Autodesk Inventor part; units mm, degrees
ref_plane "YZ Plane" through (0, 0, 0) normal (1, 0, 0) x (0, 1, 0)
ref_plane "XZ Plane" through (0, 0, 0) normal (0, 1, 0) x (-1, 0, 0)
ref_plane "XY Plane" through (0, 0, 0) normal (0, 0, 1) x (1, 0, 0)
sketch "Sketch1" plane through (0, 0, 0) normal (0, 0, 1) x (1, 0, 0)
  line L0 (63.5, 76.2) -> (0, 76.2)
  line L1 (0, 76.2) -> (0, 53.975)
  circle A0 centre (31.75, 47.625) radius 4.05
  line L2 (19.05, -6.35) -> (44.45, -6.35)
  line L3 (63.5, 53.975) -> (63.5, 76.2)
  line L4 (31.75, 76.2) -> (31.75, -6.35)
  circle A1 centre (31.75, 12.7) radius 2.6543
  circle A2 centre (31.75, -12.7) radius 2.6543
  circle A3 centre (31.75, -38.1) radius 2.6604
  line L5 (63.5, 53.975) -> (63.5, -6.35)
  line L6 (63.5, -6.35) -> (0, -6.35)
  line L7 (0, -6.35) -> (0, 53.975)
  line L8 (19.05, -15.3543) -> (19.05, -51.598)
  line L9 (19.05, -51.598) -> (44.45, -51.598)
  line L10 (44.45, -51.598) -> (44.45, -15.3543)
  line L11 (63.5, 53.975) -> (44.45, -15.3543)
  line L12 (0, 53.975) -> (19.05, -15.3543)
  point P0 (0, 0)
  dimension "d0" = 63.5
  dimension "d2" = 8.1
  dimension "d5" = 28.575
  dimension "d50" = 82.55
  dimension "d54" = 5.3086
  dimension "d55" = 63.5
  dimension "d59" = 25.4
  dimension "d60" = 25.4
  dimension "d61" = 25.4
extrude "Extrusion1" add sketch "Sketch1" along normal blind 3.302 contours L3 L11 L6 L2 L4 A1 A0 L0 | L4 A0 A1 L2 L6 L12 L1 L0 | L11 L10 L9 L8 L12 L6 L2
fillet "Fillet11" radius 17.78 1 edges at (63.5, 76.2, 1.651)
fillet "Fillet12" radius 17.78 1 edges at (0, 76.2, 1.651)
sketch "Sketch3" plane through (0, 0, 3.302) normal (0, 0, 1) x (1, 0, 0)
  circle A0 centre (31.75, 47.625) radius 4.05
  circle A1 centre (31.75, 47.625) radius 16
  circle A2 centre (31.75, 47.625) radius 8
  circle A3 centre (31.75, 47.625) radius 12
  line L0 (31.75, 47.625) -> (31.75, 69.8383)
  line L1 (31.75, 47.625) -> (53.9633, 47.625) construction
  point P0 (0, 0)
  point P1 (31.75, 59.625)
  dimension "d28" = 24
  dimension "d26" = 32
  dimension "d27" = 16
  dimension "d36" = 90
hole "Hole1" at (31.75, 59.625, 3.302) direction (0, 0, -1) diameter 4.4958 depth 14.1986 tip angle 118
pattern_circular "Circular Pattern1" count 4 over 360 about axis through (31.75, 47.625, 0) along (0, 0, 1) of "Hole1"
sketch "Sketch4" plane through (0, 0, 3.302) normal (0, 0, 1) x (1, 0, 0)
  circle A0 centre (31.75, 47.625) radius 4.05
  circle A1 centre (31.75, 47.625) radius 12
  circle A2 centre (31.75, 47.625) radius 16
  circle A3 centre (31.75, 47.625) radius 20.955
  line L0 (45.72, 76.2) -> (17.78, 76.2)
  line L1 (31.75, 47.625) -> (51.1677, 67.0427)
  line L2 (31.75, 47.625) -> (59.2107, 47.625) construction
  point P0 (0, 0)
  point P1 (46.5674, 62.4424)
  dimension "d42" = 41.91
  dimension "d40" = 24
  dimension "d41" = 32
  dimension "d58" = 45
hole "Hole2" at (46.5674, 62.4424, 3.302) direction (0, 0, -1) diameter 5.1054 depth 16.256 tip angle 118
pattern_circular "Circular Pattern2" count 4 over 360 about axis through (31.75, 47.625, 0) along (0, 0, 1) of "Hole2"
fillet "Fillet16" radius 6.35 2 edges at (44.45, -15.3543, 1.651) (19.05, -15.3543, 1.651)
sketch "Sketch5" plane through (0, 0, 3.302) normal (0, 0, 1) x (1, 0, 0)
  circle A0 centre (31.75, 47.625) radius 4.05
  circle A1 centre (31.75, 47.625) radius 7
  point P0 (0, 0)
  dimension "d64" = 14
extrude "Extrusion2" cut sketch "Sketch5" against normal blind 25.4 contours A0 | A1
equation "\"d54\" = d3"
properties part number "Arm Plate3"
Can you work these out from the model? Positions are in its coordinate system, mm. A direction names the side the tool comes from. Coordinates: 2 decimals unless noted, no trailing zeros. Order: outer loops, then holes, each group sorted by start corner. A loop starts at its lowest first (then second) coordinate and runs counter-clockwise, first axis right, second up. Notation, with made-up numbers: (86.5, 39) - (137.5, 39) arc R23 ccw to (137.5, 52) - close; hole circle Ø7 at (62, -16). An arc over 180 degrees is marked (long way). Answer in a Markdown table with one row per item.
1. If we mould it in two halves opening along X, with no side actions, what happens to faces 1 (the flat face through (32, -51.598, 2)), 2 (the cylindrical face through (34.28, -13.5, 1.63)), 3 (the flat face through (44.45, -34, 2))? For each: pulls with the +X half, pulls with the -X half, needs draft (parallel to the pull), parting line crosses it, or undercut.
Reply:
| item | result |
|---|---|
| face 1 | needs draft |
| face 2 | undercut |
| face 3 | pulls with the +X half |
2. Suppose I cut it at B-B (y = -38.1). Please give me the cut outline in (x, z).
Reply:
| item | result |
|---|---|
| outline | (19.05, 0) - (29.09, 0) - (29.09, 3.3) - (19.05, 3.3) - close; (34.41, 0) - (44.45, 0) - (44.45, 3.3) - (34.41, 3.3) - close |
3. Suppose I cut it at D-D (y = 12.7). Please give me the cut outline in (x, z).
Reply:
| item | result |
|---|---|
| outline | (11.34, 0) - (29.1, 0) - (29.1, 3.3) - (11.34, 3.3) - close; (34.4, 0) - (52.16, 0) - (52.16, 3.3) - (34.4, 3.3) - close |
4. For faces 4 (the flat face through (31, 27, 3.302)), 5 (the flat face through (19.05, -34, 2)), which set-ups out of +Z, -Z, +X, -X, +Y, -Y let a thin tool reach every point of the face, with its end or its side?
Reply:
| item | result |
|---|---|
| face 4 | +Z, +X, -X, +Y, -Y |
| face 5 | +Z, -Z, -X, -Y |
5. If I drill on line 1 along X through (y, z) = (-39.5, 0.2); line 2 along X through (y, z) = (10.5, 0.55); line 3 along Y through (x, z) = (38, 1.1), over which ranges is the centre line in solid material (lowest first)?
Reply:
| item | result |
|---|---|
| line 1 | x = 19.05 to 29.49, 34.01 to 44.45 |
| line 2 | x = 11.95 to 30.26, 33.24 to 51.55 |
| line 3 | y = -51.6 to 44.47, 50.78 to 76.2 |
6. Suppose I cut it at C-C (z = 1.1). Give the number of separate pieces and of enclosed holes in the cut face, and give its area (3 significant figures).
Reply:
| item | result |
|---|---|
| separate pieces | 1 |
| enclosed holes | 12 |
| area | 4,910 mm^2 |
7. For pin 1 (1.5 mm diameter, centred on y = 41, z = 1.5, fed in from -X), with a flat end and sliding along its axis, tell me the tip position at first contact or that it passes through.
Reply:
| item | result |
|---|---|
| pin 1 | stops at x = 3.36 |
8. Suppose I cut it at A-A (x = 31.75). Please give me the cut outline in (y, z) (3 decimals).
Reply:
| item | result |
|---|---|
| outline | (-51.598, 0) - (-40.76, 0) - (-40.76, 3.302) - (-51.598, 3.302) - close; (-35.44, 0) - (-15.354, 0) - (-15.354, 3.302) - (-35.44, 3.302) - close; (-10.046, 0) - (10.046, 0) - (10.046, 3.302) - (-10.046, 3.302) - close; (15.354, 0) - (33.377, 0) - (33.377, 3.302) - (15.354, 3.302) - close; (37.873, 0) - (40.625, 0) - (40.625, 3.302) - (37.873, 3.302) - close; (54.625, 0) - (57.377, 0) - (57.377, 3.302) - (54.625, 3.302) - close; (61.873, 0) - (76.2, 0) - (76.2, 3.302) - (61.873, 3.302) - close |
